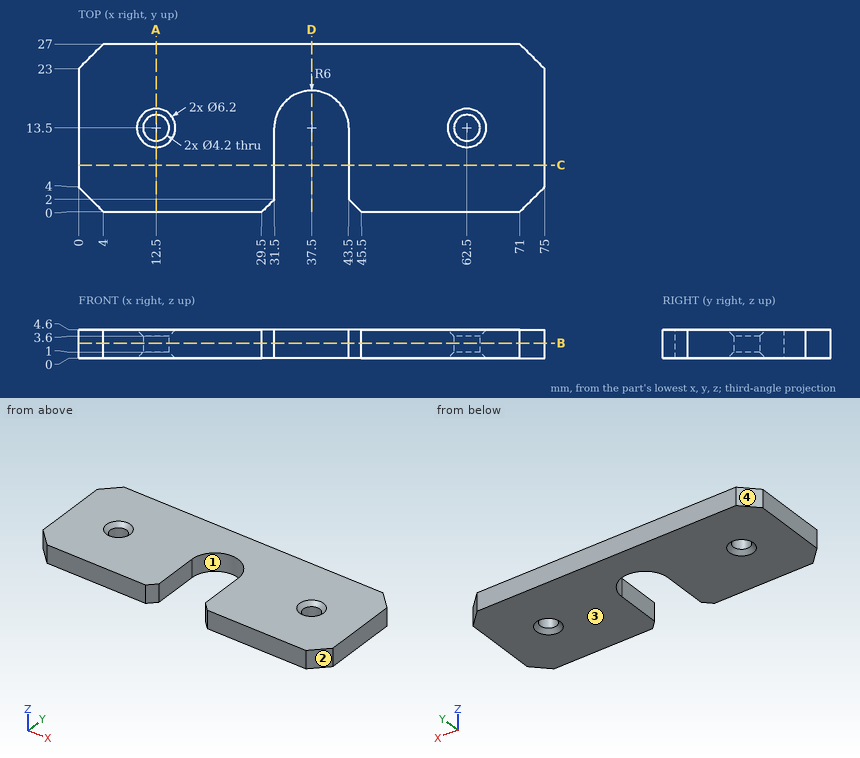
Geometry check sheet. Reference: drawing and pictorial views, mm from the part's lowest x, y, z. Round coordinates to 2 decimals unless told otherwise and drop trailing zeros. Write each loop counter-clockwise with the first axis right and the second up, starting at its lowest first coordinate (ties: lowest second). Pieces come first, ordered by that corner, then holes.
(1) Depth check by flat-ended pin: pin 1 Ø4 at (x, y) = (12.5, 13.5) entering from -Z. Enter the tip coordinate at first touch or a pass-through.
Returned:
pin 1: passes through
(2) Section check D-D (x = 37.5). Enter the section's corners in (y, z), plus the area to 3 significant figures.
Returned:
outline: (19.5, 0) - (27, 0) - (27, 4.6) - (19.5, 4.6) - close
area: 34.5 mm2
(3) Section check C-C (y = 7.5). Enter the section's corners in (x, z).
Returned:
outline: (0, 0) - (31.5, 0) - (31.5, 4.6) - (0, 4.6) - close; (43.5, 0) - (75, 0) - (75, 4.6) - (43.5, 4.6) - close
(4) Material ranges on line 1 (Y direction, x = 62.5, z = 2.7); line 2 (X direction, y = 6.5, z = 0.9); line 3 (X direction, y = 14, z = 3.65), recorded low to high.
Returned:
line 1: y = 0 to 11.4, 15.6 to 27
line 2: x = 0 to 31.5, 43.5 to 75
line 3: x = 0 to 10.41, 14.59 to 31.52, 43.48 to 60.41, 64.59 to 75
(5) Section check B-B (z = 2.45). Enter the section's corners in (x, y).
Returned:
outline: (0, 4) - (4, 0) - (29.5, 0) - (31.5, 2) - (31.5, 13.5) arc R6 cw to (43.5, 13.5) - (43.5, 2) - (45.5, 0) - (71, 0) - (75, 4) - (75, 23) - (71, 27) - (4, 27) - (0, 23) - close; hole circle Ø4.2 at (12.5, 13.5); hole circle Ø4.2 at (62.5, 13.5)
(6) Section check A-A (x = 12.5). Enter the section's corners in (y, z).
Returned:
outline: (0, 0) - (10.4, 0) - (11.4, 1) - (11.4, 3.6) - (10.4, 4.6) - (0, 4.6) - close; (15.6, 1) - (16.6, 0) - (27, 0) - (27, 4.6) - (16.6, 4.6) - (15.6, 3.6) - close
(7) Mould release check, pull along X, two halves, no side actions. Record for the marked faces 1, 2, 3 and 4: pulls with the +X half, pulls with the -X half, needs draft (parallel to the pull), parting line crosses it, or undercut.
Returned:
face 1: undercut
face 2: pulls with the +X half
face 3: needs draft
face 4: pulls with the -X half
